Geometry: see drawing. Coordinates: mm, zero at the bounding-box minimum. Round coordinates to 2 decimals unless told otherwise and drop trailing zeros. Write each loop counter-clockwise with the first axis right and the second up, starting at its lowest first coordinate (ties: lowest second). Pieces come first, ordered by that corner, then holes. Notation, with made-up numbers: M 77.5,57 L 96.5,57 A25 ccw 96.5,75 Z; hole C 31.25,25.5 d6. An arc over 180 degrees is marked long. Use one line per item in the form item = value. Start each with the question number.
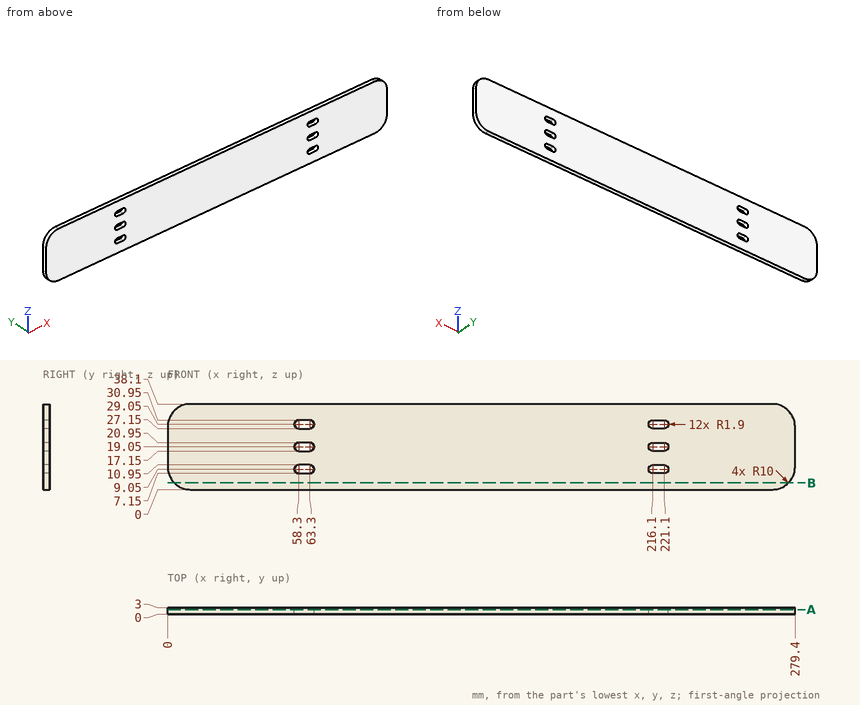
Item 1: Cut plane B-B (z = 3). Output: boundary loops of the cut face in (x, y), plus the area to 3 significant figures.
Item 2: Cut plane A-A (y = 2.1). Give the number of separate pieces and of enclosed holes in the cut face, plus the area to 3 significant figures.
Item 3: Ray query, line 1 (X direction, y = 2, z = 19.5); line 2 (X direction, y = 2.6, z = 17.5); line 3 (Z direction, x = 57, y = 0.4). Return the intervals inside material, ascending. Write a range as from..to.
Final values:
q1.outline = M 2.86,0 L 276.54,0 L 276.54,3 L 2.86,3 Z
q1.area = 821 mm^2
q2.separate_pieces = 1
q2.enclosed_holes = 6
q2.area = 10,400 mm^2
q3.line_1 = 0..56.45, 65.15..214.25, 222.95..279.4
q3.line_2 = 0..57.2, 64.4..215, 222.2..279.4
q3.line_3 = 0..7.66, 10.44..17.66, 20.44..27.66, 30.44..38.1
